from build123d import *

# Parameters (mm, degrees)
SKETCH1_W           = 35
SKETCH1_H           = 35
BOSS_EXTRUDE1_DEPTH = 5
SKETCH2_R           = 2.5
BOSS_EXTRUDE2_DEPTH = 14
FILLET1_R           = 5
CHAMFER1_SIZE       = 1
BOSS_EXTRUDE3_DEPTH = 5
SKETCH5_R           = 1.6
CUT_EXTRUDE1_DEPTH  = 14
FILLET2_R           = 5


with BuildPart() as part:
    # Sketch1 → Boss-Extrude1 (new body)
    with BuildSketch(Plane.XY):
        with Locations((17.5, -17.5)):
            Rectangle(SKETCH1_W, SKETCH1_H)
    extrude(amount=BOSS_EXTRUDE1_DEPTH)

    # Sketch2 → Boss-Extrude2 (add)
    with BuildSketch(Plane.XY.offset(5)):
        with Locations((5, -5)):
            Circle(SKETCH2_R)
        with Locations((30, -5)):
            Circle(SKETCH2_R)
        with Locations((30, -30)):
            Circle(SKETCH2_R)
        with Locations((5, -30)):
            Circle(SKETCH2_R)
    extrude(amount=BOSS_EXTRUDE2_DEPTH)

    # Fillet1
    fillet1_edges = [part.edges().sort_by_distance(p)[0] for p in [
        (0, 0, 2.5),
        (0, -35, 2.5),
        (35, -35, 2.5),
        (35, 0, 2.5),
    ]]
    fillet(fillet1_edges, radius=FILLET1_R)

    # Chamfer1
    chamfer1_edges = [part.edges().sort_by_distance(p)[0] for p in [
        (2.5, -5, 19),
        (27.5, -5, 19),
        (27.5, -30, 19),
        (2.5, -30, 19),
    ]]
    chamfer(chamfer1_edges, length=CHAMFER1_SIZE)

    # Sketch3 → Boss-Extrude3 (add)
    with BuildSketch(Plane(origin=(0, 0, 0), x_dir=(-1, 0, 0), z_dir=(0, 0, -1))):
        Polygon((-35, -30), (-35, -35), (-25, -60), (-10, -60), (0, -35), (0, -30), align=None)
    extrude(amount=-BOSS_EXTRUDE3_DEPTH)

    # Sketch5 → Cut-Extrude1 (cut)
    with BuildSketch(Plane.XY.offset(5)):
        with Locations((17.5, -55)):
            Circle(SKETCH5_R)
        with Locations((17.5, -45)):
            Circle(SKETCH5_R)
    extrude(amount=-CUT_EXTRUDE1_DEPTH, mode=Mode.SUBTRACT)

    # Fillet2
    fillet2_edges = [part.edges().sort_by_distance(p)[0] for p in [
        (35, -35, 2.5),
        (25, -60, 2.5),
        (10, -60, 2.5),
        (0, -35, 2.5),
    ]]
    fillet(fillet2_edges, radius=FILLET2_R)


solid = part.part
Geometry: final body of the model. Coordinates: model frame, mm. A direction names the side the tool comes from. Give positions to 0.01 mm unless a question says otherwise; leave off trailing zeros. Write each loop counter-clockwise with the first axis right and the second up, starting at its lowest first coordinate (ties: lowest second). Pieces come first, ordered by that corner, then holes.
(1) First-contact query: P1, Ø1.9, axis at x = 17.5, y = -55, coming from the +Z side; P2, Ø6, axis at x = 7, z = 10.5, coming from the +Y side; P3, Ø3, axis at x = 19, y = -12, coming from the +Z side; P4, Ø2, axis at x = 28, z = 7.5, coming from the +Y side. Flat tips, straight axial feed; report the tip coordinate or a pass-through.
(2) Cut plane A-A, the plane y = -45. Return loops of the section in (x, z), then the cut area to 3 significant figures.
(3) Access query for faces 5 (the cylindrical face through (7.385, -4.249, 11.409)), 6 (the cylindrical face through (33, -1, 3)). Directions: +Z, -Z, +X, -X, +Y, -Y. A direction counts if a zero-diameter tool reaches every point of the face in a straight line with its end or side. Return the directions, or none.
(4) Mould query, pull axis Y, two halves, no side actions, for faces 1 (the cylindrical face through (6.34, -27.89, 11.41)), 2 (the flat face through (4.6, -46.5, 2.5)), 3 (the flat face through (35, -19, 2)), 4 (the cylindrical face through (29.67, -27.52, 11.41)). Classes: released by +Y, released by -Y, zero draft, split by the parting line, or undercut.
(5) Cut plane C-C, the plane y = -37. Return loops of the section in (x, z).
(6) Cut plane D-D, the plane x = 24. Return loops of the section in (y, z), then the cut area to 3 significant figures.
(7) Ray query, line 1 (Y direction, x = 17.5, z = 2.4); line 2 (Y direction, x = 3, z = 11); line 3 (Z direction, x = 8.5, y = -28). Return the intervals inside material, ascending.
(8) Cut plane B-B, the plane z = 3.75. Return loops of the section in (x, y), then the cut area to 3 significant figures.
Values follow:
1. P1: passes through
1. P2: stops at y = -2.5
1. P3: stops at z = 5
1. P4: stops at y = -2.71
2. outline: (4, 0) - (15.9, 0) - (15.9, 5) - (4, 5) - close; (19.1, 0) - (31, 0) - (31, 5) - (19.1, 5) - close
2. area: 119 mm2
3. face 5: +Z
3. face 6: +Z, -Z, +X, +Y
4. face 1: undercut
4. face 2: released by -Y
4. face 3: zero draft
4. face 4: undercut
5. outline: (0.8, 0) - (34.2, 0) - (34.2, 5) - (0.8, 5) - close
6. outline: (-59.39, 0) - (0, 0) - (0, 5) - (-59.39, 5) - close
6. area: 297 mm2
7. line 1: y = -60 to -56.6, -53.4 to -46.6, -43.4 to 0
7. line 2: y = -31.5 to -28.5, -6.5 to -3.5
7. line 3: z = 0 to 5
8. outline: (0, -34.04) arc R5 ccw to (0.36, -35.89) - (8.74, -56.86) arc R5 ccw to (13.39, -60) - (21.61, -60) arc R5 ccw to (26.26, -56.86) - (34.64, -35.89) arc R5 ccw to (35, -34.04) - (35, -5) arc R5 ccw to (30, 0) - (5, 0) arc R5 ccw to (0, -5) - close; hole circle Ø3.2 at (17.5, -55); hole circle Ø3.2 at (17.5, -45)
8. area: 1,820 mm2
